Work out the finished part from the listing and answer in its coordinate system (mm). A direction names the side the tool comes from. Coordinates: 2 decimals unless noted, no trailing zeros. Order: outer loops, then holes, each group sorted by start corner. A loop starts at its lowest first (then second) coordinate and runs counter-clockwise, first axis right, second up. Notation, with made-up numbers: (54.5, -18.5) -> (102.5, -18.5) arc R34 cw to (102.5, 11.5) -> close; hole circle Ø5 at (-14.75, 83). An arc over 180 degrees is marked (long way). Write item = value, one per line. Start each with the question number.
Q1. Which of the six approach directions +Z, -Z, +X, -X, +Y, -Y give full straight-line access (tool end or side, diameter ignored) to faces 4 (the flat face through (-61, 0, -8)), 5 (the flat face through (60, 0, -8)), 6 (the flat face through (0, -5, -8))?
Q2. The part is cut by section D-D, the plane z = -30.5. Determine the outline of the cut face in (x, y), plus the area to 3 significant figures.
Q3. The part is cut by section B-B, the plane z = -13. Determine the outline of the cut face in (x, y), plus the area to 3 significant figures.
Q4. Straight lines are drawn through the part: L1, parallel to Y at x = 2, z = -48; L2, parallel to X at y = -1.25, z = -57.5; L3, parallel to Y at x = 58.5, z = -1. For each, find the intervals that lie inside material, in ascending order. Write a range as from..to.
Q5. The part is cut by section A-A, the plane x = -81. Determine the outline of the cut face in (y, z), plus the area to 3 significant figures.
Q6. For a pull along Y with two mould halves and no side action, classify faces 1 (the flat face through (-94.958, 10.761, 5.046)), 2 (the flat face through (14.25, 0.04, -14.08)), 3 (the cylindrical face through (0, 0, -46)) as +Y half, -Y half, draft (parallel to the pull), parting line (faces both ways), or undercut.
Q7. Flat-ended cylindrical pins translate along their axes: pin 1 (3.5 mm diameter, centred on y = 12.86, z = 15.32, fed in from -X); pin 2 (3 mm diameter, centred on y = -3.5, z = -35, fed in from +X); pin 3 (6 mm diameter, centred on x = 1, z = -14, fed in from +Y); pin 4 (2 mm diameter, centred on y = -4, z = -40.5, fed in from -X). Find the tip coordinate at first contact, or state that the pin passes through.
Q8. The part is cut by section C-C, the plane x = -14.5. Determine the outline of the cut face in (y, z).
```python
from build123d import *

# Parameters (mm, degrees)
EXTRUDE_1_DEPTH          = 5
FILLET_1_R               = 5
EXTRUDE_START            = 98
SKETCH_9_R               = 1.563633766
EXTRUDE_4_DEPTH          = 6
EXTRUDE_START_2          = -92
SKETCH_9_2_R             = 1.563633766
EXTRUDE_5_DEPTH          = 6
SKETCH_10_R              = 2
EXTRUDE_6_DEPTH          = 4
CUT_EXTRUDE_1_DEPTH      = 131.654334604
CUT_EXTRUDE_1_DEPTH_BACK = 131.654334604
SKETCH_11_R              = 2
CHAMFER_1_SIZE           = 2


with BuildPart() as part:
    # 草图1 → 凸台-拉伸1 (new, symmetric)
    with BuildSketch(Plane(origin=(0, 0, 0), x_dir=(1, 0, 0), z_dir=(0, 1, 0))):
        Polygon((98, 0), (-98, 0), (-98, 8), (-24.784609691, 8), (-4, 20), (-4, 55), (4, 55), (4, 20), (24.784609691, 8), (98, 8), align=None)
    extrude(amount=EXTRUDE_1_DEPTH, both=True)

    # 圆角1
    fillet_1_edges = [part.edges().sort_by_distance(p)[0] for p in [
        (0, -5, -55),
        (0, 5, -55),
    ]]
    fillet(fillet_1_edges, radius=FILLET_1_R - 0.0001)  # a hair under: the kernel refuses the full size

    # 草图9 → 凸台-拉伸4 (add)
    with BuildSketch(Plane(origin=(0, 0, 0), x_dir=(0, 0, -1), z_dir=(1, 0, 0)).offset(EXTRUDE_START)):
        with BuildLine():
            Line((3.213938048, 3.830222216), (-12.106950814, 16.685974409))
            ThreePointArc((-12.106950814, 16.685974409), (-19.151111078, 16.069690242), (-18.534826911, 9.025529978))
            Line((-18.534826911, 9.025529978), (-3.213938048, -3.830222216))
            ThreePointArc((-3.213938048, -3.830222216), (3.830222216, -3.213938048), (3.213938048, 3.830222216))
        make_face()
        with Locations(Location((-15.320888862, 12.855752194, 0), (0, 0, 180))):
            Circle(SKETCH_9_R, mode=Mode.SUBTRACT)
    extrude(amount=-EXTRUDE_4_DEPTH)

    # 草图9<2> → 凸台-拉伸5 (add)
    with BuildSketch(Plane(origin=(0, 0, 0), x_dir=(0, 0, -1), z_dir=(1, 0, 0)).offset(EXTRUDE_START_2)):
        with BuildLine():
            Line((3.213938048, 3.830222216), (-12.106950814, 16.685974409))
            ThreePointArc((-12.106950814, 16.685974409), (-19.151111078, 16.069690242), (-18.534826911, 9.025529978))
            Line((-18.534826911, 9.025529978), (-3.213938048, -3.830222216))
            ThreePointArc((-3.213938048, -3.830222216), (3.830222216, -3.213938048), (3.213938048, 3.830222216))
        make_face()
        with Locations(Location((-15.320888862, 12.855752194, 0), (0, 0, 180))):
            Circle(SKETCH_9_2_R, mode=Mode.SUBTRACT)
    extrude(amount=-EXTRUDE_5_DEPTH)

    # 草图10 → 凸台-拉伸6 (add, symmetric)
    with BuildSketch(Plane(origin=(0, 0, 0), x_dir=(0, 0, -1), z_dir=(1, 0, 0))):
        with BuildLine():
            Line((50.868240888, 4.924038765), (80.412473479, -0.285406565))
            ThreePointArc((80.412473479, -0.285406565), (84.468271355, -6.077686218), (78.675991702, -10.133484095))
            Line((78.675991702, -10.133484095), (49.131759112, -4.924038765))
            ThreePointArc((49.131759112, -4.924038765), (45.075961235, 0.868240888), (50.868240888, 4.924038765))
        make_face()
        with Locations((79.54423259, -5.20944533)):
            Circle(SKETCH_10_R, mode=Mode.SUBTRACT)
    extrude(amount=EXTRUDE_6_DEPTH, both=True)

    # 草图11 → 切除-拉伸1 (cut, two sides: drawn at the far end of the back side and taken through both)
    with BuildSketch(Plane(origin=(0, 0, 0), x_dir=(0, 0, -1), z_dir=(1, 0, 0)).offset(-CUT_EXTRUDE_1_DEPTH_BACK)):
        with Locations((48, 0)):
            Circle(SKETCH_11_R)
    extrude(amount=CUT_EXTRUDE_1_DEPTH + CUT_EXTRUDE_1_DEPTH_BACK, mode=Mode.SUBTRACT)

    # 倒角1
    chamfer_1_edges = [part.edges().sort_by_distance(p)[0] for p in [
        (-61.392304845, -5, -8),
        (-14.392304845, -5, -14),
        (14.392304845, -5, -14),
        (61.392304845, -5, -8),
        (61.392304845, 5, -8),
        (-98, 0, -8),
        (98, 0, -8),
        (14.392304845, 5, -14),
        (-14.392304845, 5, -14),
        (-61.392304845, 5, -8),
    ]]
    chamfer(chamfer_1_edges, length=CHAMFER_1_SIZE)


solid = part.part
```
Model answer:
q1.face_4 = -Z, -X, +Y, -Y
q1.face_5 = -Z, +X, +Y, -Y
q1.face_6 = +Z, +X, -X, -Y
q2.outline = (-4, -5) -> (4, -5) -> (4, 5) -> (-4, 5) -> close
q2.area = 80.0 mm2
q3.outline = (-16.12, -3) -> (-12.12, -5) -> (12.12, -5) -> (16.12, -3) -> (16.12, 3) -> (12.12, 5) -> (-12.12, 5) -> (-16.12, 3) -> close
q3.area = 306 mm2
q4.L1 = -5..-2, 2..5
q4.L2 = -4..4
q4.L3 = -5..5
q5.outline = (-5, -6) -> (-3, -8) -> (3, -8) -> (5, -6) -> (5, 0) -> (-5, 0) -> close
q5.area = 76.0 mm2
q6.face_1 = +Y half
q6.face_2 = draft
q6.face_3 = undercut
q7.pin_1 = -98
q7.pin_2 = 4
q7.pin_3 = 5
q7.pin_4 = -4
q8.outline = (-5, -11.63) -> (-3, -13.94) -> (3, -13.94) -> (5, -11.63) -> (5, 0) -> (-5, 0) -> close
